Geometry: final body of the model. Coordinates: model frame, mm. Face numbers are marked on the shaded views. A direction names the side the tool comes from. Coordinates: 2 decimals unless noted, no trailing zeros. Order: outer loops, then holes, each group sorted by start corner. A loop starts at its lowest first (then second) coordinate and runs counter-clockwise, first axis right, second up. Notation, with made-up numbers: (53, 72.25) -> (95, 72.25) arc R10 cw to (95, 82.25) -> close; hole circle Ø6 at (17, -14.5). An arc over 180 degrees is marked (long way). Answer in a Markdown table with one row per item. Add a question column.
1) Contact query for flat-ended pins moving along their axis: P1, Ø6.5, axis at x = 241.5, y = 7.5, coming from the -Z side (3 decimals); P2, Ø2, axis at x = 75, z = -35.5, coming from the +Y side (3 decimals). Output: stop coordinate, or through.
2) Set-up query: the marked faces 1 and 2. Return all of +Z, -Z, +X, -X, +Y, -Y with unobstructed straight access to the full face (end or side cutting, diameter ignored); none if empty.
3) Ray query, line 1 (Z direction, x = 138, y = 3.75) (3 decimals); line 2 (Y direction, x = 200.5, z = -8.5) (3 decimals); line 3 (Y direction, x = 60, z = -2.5). Return the intervals inside material, ascending. Write a range as from..to.
4) Section query B-B on x = 415. Return the cut outline in (y, z) (3 decimals).
5) Section query C-C on y = 9.25. Return the cut outline in (x, z) (3 decimals), then the cut area to 3 significant figures.
6) Section query A-A on z = -34. Return the cut outline in (x, y) (3 decimals), then the cut area to 3 significant figures.
```python
from build123d import *

# Parameters (mm, degrees)
SKETCH1_W           = 50.8
SKETCH1_H           = 12.13231
BOSS_EXTRUDE1_DEPTH = 457.2
CUT_EXTRUDE1_DEPTH  = 457.2


with BuildPart() as part:
    # Sketch1 → Boss-Extrude1 (new body)
    with BuildSketch(Plane(origin=(0, 0, 0), x_dir=(0, 0, -1), z_dir=(1, 0, 0))):
        with Locations((25.4, 6.066155)):
            Rectangle(SKETCH1_W, SKETCH1_H)
    extrude(amount=BOSS_EXTRUDE1_DEPTH)

    # Sketch2 → Cut-Extrude1 (cut)
    with BuildSketch(Plane.ZY):
        Polygon((-41.275, 12.13231), (-3.175, 12.13231), (0, 12.13231), (-3.175, 11.572471836), (-3.175, 3.175), (-41.275, 3.175), (-50.8, 3.175), (-50.8, 12.13231), align=None)
    extrude(amount=-CUT_EXTRUDE1_DEPTH, mode=Mode.SUBTRACT)


solid = part.part
```
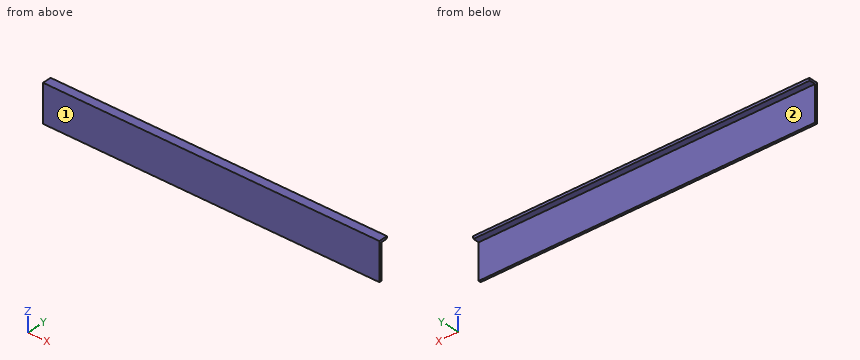
Result:
| question | item | result |
|---|---|---|
| 1 | P1 | z = -3.175 |
| 1 | P2 | y = 3.175 |
| 2 | face 1 | +Z, -Z, +X, -X, -Y |
| 2 | face 2 | -Z, +X, -X, +Y |
| 3 | line 1 | -3.175..0 |
| 3 | line 2 | 0..3.175 |
| 3 | line 3 | 0..11.69 |
| 4 | outline | (0, -50.8) -> (3.175, -50.8) -> (3.175, -3.175) -> (11.572, -3.175) -> (12.132, 0) -> (0, 0) -> close |
| 5 | outline | (0, -3.175) -> (457.2, -3.175) -> (457.2, 0) -> (0, 0) -> close |
| 5 | area | 1,450 mm2 |
| 6 | outline | (0, 0) -> (457.2, 0) -> (457.2, 3.175) -> (0, 3.175) -> close |
| 6 | area | 1,450 mm2 |
